Autodesk Inventor part; units mm, degrees
ref_plane "YZ Plane" through (0, 0, 0) normal (1, 0, 0) x (0, 1, 0)
ref_plane "XZ Plane" through (0, 0, 0) normal (0, 1, 0) x (-1, 0, 0)
ref_plane "XY Plane" through (0, 0, 0) normal (0, 0, 1) x (1, 0, 0)
sketch "Sketch1" plane through (0, 0, 0) normal (0, 0, 1) x (1, 0, 0)
  line L0 (100.4457, -5.6676) -> (100.4457, -66.5884)
  line L1 (75.0457, -66.5884) -> (75.0457, -5.6676)
  line L2 (75.0457, -5.6676) -> (55.9957, -5.6676)
  line L3 (55.9957, -5.6676) -> (55.9957, -66.5884)
  line L4 (55.9957, -66.5884) -> (75.0457, -66.5884)
  line L5 (75.0457, -66.5884) -> (75.0457, -5.6676)
  line L6 (75.0457, -5.6676) -> (62.3457, -5.6676)
  line L7 (62.3457, -5.6676) -> (62.3457, -66.5884)
  line L8 (62.3457, -66.5884) -> (75.0457, -66.5884)
  line L9 (75.0457, -66.5884) -> (75.0457, -5.6676)
  line L10 (55.9957, -5.6676) -> (59.1707, -5.6676)
  line L11 (59.1707, -5.6676) -> (59.1707, -66.5884)
  line L12 (59.1707, -5.6676) -> (59.1707, -12.0176)
  circle A0 centre (59.1707, -12.0176) radius 1.5
  line L13 (59.1707, -66.5884) -> (59.1707, -60.2384)
  circle A1 centre (59.1707, -60.2384) radius 1.5
  line L14 (59.1707, -12.0176) -> (59.1707, -36.1222)
  circle A2 centre (59.1707, -36.1222) radius 1.5
  point P0 (0, 0)
  dimension "d0" = 19.05
  dimension "d1" = 12.7
  dimension "d2" = 3.175
  dimension "d3" = 6.35
  dimension "d4" = 3
  dimension "d5" = 6.35
  dimension "d6" = 3
  dimension "d7" = 24.1046
  dimension "d8" = 3
extrude "Extrusion1" add sketch "Sketch1" along normal blind 12.7
sketch "Sketch2" plane through (75.0457, -66.5884, 0) normal (1, 0, 0) x (0, 0, -1)
  line L0 (0, 60.9208) -> (0, 0)
  line L1 (0, 0) -> (0, 30.4546)
  line L2 (0, 30.4546) -> (-6.35, 30.4546)
  circle A0 centre (-6.35, 30.4546) radius 3.95
  point P0 (0, 66.5884)
  dimension "d11" = 30.4546
  dimension "d12" = 6.35
  dimension "d13" = 7.9
extrude "Extrusion2" add sketch "Sketch2" along normal blind 19.05
sketch "Sketch3" plane through (0, 0, 12.7) normal (0, 0, 1) x (1, 0, 0)
  line L0 (75.0457, -5.6676) -> (55.9957, -5.6676)
  line L1 (55.9957, -5.6676) -> (55.9957, -66.5884)
  line L2 (55.9957, -66.5884) -> (75.0457, -66.5884)
  line L3 (75.0457, -5.6676) -> (62.3457, -5.6676)
  line L4 (62.3457, -5.6676) -> (62.3457, -66.5884)
  line L5 (62.3457, -66.5884) -> (75.0457, -66.5884)
  line L6 (55.9957, -5.6676) -> (59.1707, -5.6676)
  line L7 (59.1707, -5.6676) -> (59.1707, -66.5884)
  line L8 (59.1707, -5.6676) -> (59.1707, -12.0176)
  circle A0 centre (59.1707, -12.0176) radius 1.5
  line L9 (59.1707, -66.5884) -> (59.1707, -60.2384)
  circle A1 centre (59.1707, -60.2384) radius 1.5
  line L10 (59.1707, -12.0176) -> (59.1707, -36.1222)
  circle A2 centre (59.1707, -36.1222) radius 1.5
  line L11 (55.9957, -5.6676) -> (62.3457, -5.6676)
  line L12 (62.3457, -5.6676) -> (62.3457, -66.5884)
  line L13 (62.3457, -66.5884) -> (55.9957, -66.5884)
  line L14 (55.9957, -66.5884) -> (55.9957, -5.6676)
  line L15 (75.0457, -66.5884) -> (75.0457, -5.6676)
  line L16 (62.3457, -5.6676) -> (75.0457, -5.6676)
  line L17 (75.0457, -5.6676) -> (75.0457, -12.0176)
  line L18 (75.0457, -12.0176) -> (62.3457, -12.0176)
  line L19 (62.3457, -12.0176) -> (62.3457, -5.6676)
  line L20 (62.3457, -66.5884) -> (75.0457, -66.5884)
  line L21 (75.0457, -66.5884) -> (75.0457, -60.2384)
  line L22 (75.0457, -60.2384) -> (62.3457, -60.2384)
  line L23 (62.3457, -60.2384) -> (62.3457, -66.5884)
  point P0 (0, 0)
  dimension "d16" = 19.05
  dimension "d17" = 12.7
  dimension "d18" = 3.175
  dimension "d19" = 6.35
  dimension "d20" = 3
  dimension "d21" = 6.35
  dimension "d22" = 3
  dimension "d23" = 24.1046
  dimension "d24" = 3
  dimension "d27" = 60.9208
  dimension "d28" = 6.35
  dimension "d29" = 6.35
extrude "Extrusion3" cut sketch "Sketch3" against normal blind 2540 contours L15 L18 L4 L0 | L4 L2 L7 A1 A2 A0 L0 | L7 A0 A2 A1 L2 L1 L0 | L15 L2 L4 L22 | A0 L7 | L7 A0 | A2 L7 | L7 A2 | A1 L7 | L7 A1
fillet "Fillet1" radius 1 8 edges at (62.3457, -36.128, 12.7) (75.0457, -36.128, 12.7) (68.6957, -60.2384, 12.7) (68.6957, -12.0176, 12.7) (62.3457, -12.0176, 6.35) (62.3457, -60.2384, 6.35) (75.0457, -60.2384, 6.35) (75.0457, -12.0176, 6.35)
fillet "Fillet2" radius 1 1 edges at (94.0957, -36.1338, 10.3)
fillet "Fillet3" [suppressed]
sketch "Sketch5" plane through (0, 0, 0) normal (0, 0, -1) x (-1, 0, 0)
  line L0 (-63.3457, -12.0176) -> (-74.0457, -12.0176)
  line L1 (-74.0457, -12.0176) -> (-72.0457, -12.0176)
  line L2 (-72.0457, -12.0176) -> (-72.0457, -15.0176)
  circle A0 centre (-72.0457, -15.0176) radius 1.25
  line L3 (-68.6957, -12.0176) -> (-68.6957, -9.3578)
  line L4 (-62.3457, -59.2384) -> (-62.3457, -13.0176)
  line L5 (-62.3457, -36.128) -> (-58.1504, -36.128)
  line L6 (-74.0457, -12.0176) -> (-63.3457, -12.0176)
  line L7 (-63.3457, -12.0176) -> (-65.3457, -12.0176)
  line L8 (-65.3457, -12.0176) -> (-65.3457, -15.0176)
  circle A1 centre (-65.3457, -15.0176) radius 1.25
  line L9 (-72.0457, -60.2384) -> (-72.0457, -57.2384)
  circle A2 centre (-72.0457, -57.2384) radius 1.25
  line L10 (-65.3457, -60.2384) -> (-65.3457, -57.2384)
  circle A3 centre (-65.3457, -57.2384) radius 1.25
  point P0 (0, 0)
  dimension "d48" = 2
  dimension "d49" = 3
  dimension "d50" = 2.5
extrude "Extrusion5" cut sketch "Sketch5" against normal blind 9
properties part number "BackWheelMount"
Check sheet for the modelled part. Datum: model origin and axes. Units: mm. A direction names the side the tool comes from. Coordinates: 2 decimals unless noted, no trailing zeros. Order: outer loops, then holes, each group sorted by start corner. A loop starts at its lowest first (then second) coordinate and runs counter-clockwise, first axis right, second up. Notation, with made-up numbers: M 73,16 L 79,16 A25 ccw 79,28 Z; hole C 87.5,1 d3. An arc over 180 degrees is marked long. One line per question, with ' | ' between items. Start each with the question number.
Item 1: Material ranges on line 1 (X direction, y = -15.5, z = 3); line 2 (X direction, y = -44, z = 5); line 3 (Y direction, x = 65, z = 3.5), recorded low to high.
Item 2: Sectioned sample at D-D on z = 8.5. Count the separate pieces of the cut face and the enclosed holes in it, and give its area (3 significant figures).
Item 3: Sectioned sample at C-C on x = 86. Record the cut outline in (y, z), and give its area (3 significant figures).
Item 4: Gauge pin test, flat ends, axial feed: P1, Ø6, axis at x = 78.5, z = 2, coming from the -Y side; P2, Ø4, axis at x = 81.5, z = 6, coming from the -Y side; P3, Ø6, axis at y = -53, z = 8.5, coming from the +X side. Record the tip position at first contact, or that the pin passes through.
Item 5: Mould release check, pull along Y, two halves, no side actions. Record for faces 3 (the cylindrical face through (62.646, -36.452, 12.415)), 4 (the flat face through (72, -15, 9)), 5 (the cylindrical face through (62.63, -12.32, 5.77)): pulls with the +Y half, pulls with the -Y half, needs draft (parallel to the pull), parting line crosses it, or undercut.
Item 6: Access from +Z, -Z, +X, -X, +Y, -Y to the whole of each face (thin tool, end or side, straight path). Record for faces 1 (the cylindrical face through (64.77, -58.35, 4.44)), 2 (the cylindrical face through (75, -36, 12)).
Item 7: Sectioned sample at B-B on z = 6.35. Record the cut outline in (x, y).
Item 8: Sectioned sample at A-A on y = -30.5. Record the cut outline in (x, z), and give its area (3 significant figures).
Answer below:
1) line 1: x = 62.35 to 64.19, 66.5 to 70.89, 73.2 to 75.05 | line 2: x = 62.35 to 75.05 | line 3: y = -60.24 to -58.44, -56.04 to -16.22, -13.82 to -12.02
2) separate pieces: 1 | enclosed holes: 4 | area: 718 mm^2
3) outline: C -36.13,6.35 d7.9 | area: 49.0 mm^2
4) P1: stops at y = -39.85 | P2: stops at y = -40.08 | P3: stops at x = 75.05
5) face 3: needs draft | face 4: undercut | face 5: pulls with the +Y half
6) face 1: -Z | face 2: +Z, +X, +Y, -Y
7) outline: M 62.35,-59.24 A1 ccw 63.35,-60.24 L 74.05,-60.24 A1 ccw 75.05,-59.24 L 75.05,-40.08 L 93.1,-40.08 A1 ccw 94.1,-39.08 L 94.1,-33.18 A1 ccw 93.1,-32.18 L 75.05,-32.18 L 75.05,-13.02 A1 ccw 74.05,-12.02 L 63.35,-12.02 A1 ccw 62.35,-13.02 Z; hole C 65.35,-57.24 d2.5; hole C 65.35,-15.02 d2.5; hole C 72.05,-57.24 d2.5; hole C 72.05,-15.02 d2.5
8) outline: M 62.35,0 L 75.05,0 L 75.05,11.7 A1 ccw 74.05,12.7 L 63.35,12.7 A1 ccw 62.35,11.7 Z | area: 161 mm^2
